Source: CAD feature listing. Evaluate the final solid. Frame: model axes, mm. Coordinates: 2 decimals unless noted, no trailing zeros. Write each loop counter-clockwise with the first axis right and the second up, starting at its lowest first coordinate (ties: lowest second). Pieces come first, ordered by that corner, then holes. Notation, with made-up numbers: (29.25, 5) -> (42.25, 5) arc R14 cw to (42.25, 18) -> close; hole circle Ø1 at (81.5, 24). An arc over 180 degrees is marked (long way). Write item = value, one per line.
from build123d import *

# Parameters (mm, degrees)
SKETCH_1_R         = 8
EXTRUDE_1_DEPTH    = 8
SKETCH_2_R         = 14
SKETCH_2_R_2       = 8
EXTRUDE_2_DEPTH    = 8
HOLE_WIZARD_M5_1_D = 5.5


with BuildPart() as part:
    # 草图1 → 凸台-拉伸1 (new body)
    with BuildSketch(Plane(origin=(0, 0, 0), x_dir=(1, 0, 0), z_dir=(0, 1, 0))):
        with BuildLine():
            Line((-25, 4.45481098), (-25, -4.54518902))
            Line((-25, -4.54518902), (-5.499282233, -12.874699799))
            ThreePointArc((-5.499282233, -12.874699799), (0, -14), (5.499282233, -12.874699799))
            Line((5.499282233, -12.874699799), (25, -4.54518902))
            Line((25, -4.54518902), (25, 4.45481098))
            Line((25, 4.45481098), (5.549682792, 12.853054925))
            ThreePointArc((5.549682792, 12.853054925), (0, 14), (-5.549682792, 12.853054925))
            Line((-5.549682792, 12.853054925), (-25, 4.45481098))
        make_face()
        with Locations(Location((0, 0, 0), (0, 0, 270))):
            Circle(SKETCH_1_R, mode=Mode.SUBTRACT)
    extrude(amount=EXTRUDE_1_DEPTH)

    # 草图2 → 凸台-拉伸2 (add)
    with BuildSketch(Plane(origin=(0, 8, 0), x_dir=(1, 0, 0), z_dir=(0, 1, 0))):
        with Locations(Location((0, 0, 0), (0, 0, 113.353686186))):
            Circle(SKETCH_2_R)
        with Locations(Location((0, 0, 0), (0, 0, 270))):
            Circle(SKETCH_2_R_2, mode=Mode.SUBTRACT)
    extrude(amount=EXTRUDE_2_DEPTH)

    # M5 间隙孔1 (through all)
    with Locations(Plane(origin=(0, 8, 0), x_dir=(1, 0, 0), z_dir=(0, 1, 0))):
        with Locations((-20, 0), (20, 0)):
            Hole(HOLE_WIZARD_M5_1_D / 2)


solid = part.part
1) Cut plane A-A, the plane z = 0. Output: boundary loops of the cut face in (x, y), and give its area (3 significant figures).
Answer block:
outline = (-25, 0) -> (-22.75, 0) -> (-22.75, 8) -> (-25, 8) -> close; (-17.25, 0) -> (-8, 0) -> (-8, 16) -> (-14, 16) -> (-14, 8) -> (-17.25, 8) -> close; (8, 0) -> (17.25, 0) -> (17.25, 8) -> (14, 8) -> (14, 16) -> (8, 16) -> close; (22.75, 0) -> (25, 0) -> (25, 8) -> (22.75, 8) -> close
area = 280 mm2
2) Cut plane C-C, the plane y = 7.5. Output: boundary loops of the cut face in (x, z), and give its area (3 significant figures).
Answer block:
outline = (-25, -4.45) -> (-5.55, -12.85) arc R14 ccw to (5.55, -12.85) -> (25, -4.45) -> (25, 4.55) -> (5.5, 12.87) arc R14 ccw to (-5.5, 12.87) -> (-25, 4.55) -> close; hole circle Ø5.5 at (-20, 0); hole circle Ø16 at (0, 0); hole circle Ø5.5 at (20, 0)
area = 729 mm2
3) Cut plane B-B, the plane x = 0. Output: boundary loops of the cut face in (y, z).
Answer block:
outline = (0, -14) -> (16, -14) -> (16, -8) -> (0, -8) -> close; (0, 8) -> (16, 8) -> (16, 14) -> (0, 14) -> close
4) First-contact query: pin 1 Ø13 at (x, z) = (0, 0) entering from -Y; pin 2 Ø8 at (x, y) = (-7, 12) entering from +Z; pin 3 Ø12 at (x, z) = (19.5, 8.5) entering from +Y; pin 4 Ø5 at (y, z) = (12, -10.5) entering from -X. Flat tips, straight axial feed; report the tip coordinate or a pass-through.
Answer block:
pin_1 = through
pin_2 = 13.67
pin_3 = 8
pin_4 = -11.49
5) Material intervals for probe 1 along Y at (x, z) = (11.5, -9.25); probe 2 along X at (y, z) = (10.5, -6.5); probe 3 along X at (y, z) = (10.25, 0), sorted ascending. Write a range as [from, to].
Answer block:
probe_1 = [0, 8]
probe_2 = [-12.4, -4.66], [4.66, 12.4]
probe_3 = [-14, -8], [8, 14]
6) Cut plane D-D, the plane z = -3.25. Output: boundary loops of the cut face in (x, y), and give its area (3 significant figures).
Answer block:
outline = (-25, 0) -> (-7.31, 0) -> (-7.31, 16) -> (-13.62, 16) -> (-13.62, 8) -> (-25, 8) -> close; (7.31, 0) -> (25, 0) -> (25, 8) -> (13.62, 8) -> (13.62, 16) -> (7.31, 16) -> close
area = 384 mm2
7) Pull-direction query (X, two-part tool) for faces 1 (the flat face through (-15.14, 3.94, -8.71)), 2 (the flat face through (17, 8, 1)), 3 (the flat face through (15.11, 3.94, 8.77)), 4 (the cylindrical face through (22.747, 3.944, -0.121)); classes: +X half, -X half, draft (parallel to the pull), parting line (faces both ways), or undercut.
Answer block:
face_1 = -X half
face_2 = draft
face_3 = +X half
face_4 = undercut
